Geometry: final body of the model. Coordinates: model frame, mm. A direction names the side the tool comes from. Round coordinates to 2 decimals unless told otherwise and drop trailing zeros. Loops run counter-clockwise (first coordinate to the right, second up) from the corner with the lowest first, then second, coordinate; pieces in that order, holes last. Notation, with made-up numbers: (-19.75, 70) -> (26.25, 70) arc R22 ccw to (26.25, 99) -> close; hole circle Ø10 at (-6.5, 37). An arc over 180 degrees is marked (long way). Answer in a Markdown table with one row per item.
```python
from build123d import *

# Parameters (mm, degrees)
ESQUISSE1_R             = 1.1
BOSS_EXTRU_1_DEPTH      = 2.1
ESQUISSE2_R             = 3.35
ESQUISSE2_R_2           = 2.55
BOSS_EXTRU_2_DEPTH      = 0.2
ENL_V_START             = -0.8
ESQUISSE9_R             = 2.55
ENL_V_MAT_EXTRU_4_DEPTH = 0.8
BOSS_EXTRU_3_START      = 2.5
ESQUISSE5_R             = 3.35
ESQUISSE5_R_2           = 2.55
BOSS_EXTRU_3_DEPTH      = 4.8
ENL_V_MAT_EXTRU_3_REACH = 26.785
ESQUISSE7_R             = 0.5


with BuildPart() as part:
    # Esquisse1 → Boss.-Extru.1 (new body)
    with BuildSketch(Plane(origin=(0, 0, 0), x_dir=(1, 0, 0), z_dir=(0, 1, 0))):
        with BuildLine():
            Line((8.85, 1.9), (-5.55, 3.193286234))
            Line((-5.55, 3.193286234), (-5.55, 6.3))
            ThreePointArc((-5.55, 6.3), (-7.4, 8.15), (-9.25, 6.3))
            Line((-9.25, 6.3), (-9.25, 2.95))
            Line((-9.25, 2.95), (-21.15, 1.8))
            ThreePointArc((-21.15, 1.8), (-22.95, 0), (-21.15, -1.8))
            Line((-21.15, -1.8), (-9.25, -2.95))
            Line((-9.25, -2.95), (-9.25, -6.3))
            ThreePointArc((-9.25, -6.3), (-7.4, -8.15), (-5.55, -6.3))
            Line((-5.55, -6.3), (-5.55, -3.193286234))
            Line((-5.55, -3.193286234), (8.85, -1.9))
            ThreePointArc((8.85, -1.9), (10.75, 0), (8.85, 1.9))
        make_face()
        with Locations(Location((-7.4, 0, 0), (0, 0, 270))):
            Circle(ESQUISSE1_R, mode=Mode.SUBTRACT)
    extrude(amount=BOSS_EXTRU_1_DEPTH)

    # Esquisse2 → Boss.-Extru.2 (add)
    with BuildSketch(Plane(origin=(0, 2.1, 0), x_dir=(1, 0, 0), z_dir=(0, 1, 0))):
        with Locations(Location((-7.4, 0, 0), (0, 0, 270))):
            Circle(ESQUISSE2_R)
        with Locations(Location((-7.4, 0, 0), (0, 0, 270))):
            Circle(ESQUISSE2_R_2, mode=Mode.SUBTRACT)
    extrude(amount=BOSS_EXTRU_2_DEPTH)

    # Esquisse9 → Enlèv. mat.-Extru.4 (cut)
    with BuildSketch(Plane(origin=(0, 2.3, 0), x_dir=(1, 0, 0), z_dir=(0, 1, 0)).offset(ENL_V_START)):
        with Locations(Location((-7.4, 0, 0), (0, 0, 270))):
            Circle(ESQUISSE9_R)
    extrude(amount=ENL_V_MAT_EXTRU_4_DEPTH, mode=Mode.SUBTRACT)

    # Esquisse5 → Boss.-Extru.3 (add)
    with BuildSketch(Plane.XZ.offset(BOSS_EXTRU_3_START)):
        with Locations(Location((-7.4, 0, 0), (0, 0, 90))):
            Circle(ESQUISSE5_R)
        with Locations(Location((-7.4, 0, 0), (0, 0, 90))):
            Circle(ESQUISSE5_R_2, mode=Mode.SUBTRACT)
    extrude(amount=-BOSS_EXTRU_3_DEPTH)

    # Esquisse7 → Enlèv. mat.-Extru.3 (cut, up to next)
    with BuildSketch(Plane(origin=(0, 2.1, 0), x_dir=(1, 0, 0), z_dir=(0, 1, 0)), mode=Mode.PRIVATE) as enl_v_mat_extru_3_sk1:
        with Locations(Location((-7.4, 4.35, 0), (0, 0, 270))):
            Circle(ESQUISSE7_R)
    enl_v_mat_extru_3_tool1 = extrude(enl_v_mat_extru_3_sk1.sketch, amount=-ENL_V_MAT_EXTRU_3_REACH, mode=Mode.PRIVATE) & part.part
    # Esquisse7 → Enlèv. mat.-Extru.3 (cut, up to next)
    with BuildSketch(Plane(origin=(0, 2.1, 0), x_dir=(1, 0, 0), z_dir=(0, 1, 0)), mode=Mode.PRIVATE) as enl_v_mat_extru_3_sk2:
        with Locations(Location((-7.4, 6.65, 0), (0, 0, 270))):
            Circle(ESQUISSE7_R)
    enl_v_mat_extru_3_tool2 = extrude(enl_v_mat_extru_3_sk2.sketch, amount=-ENL_V_MAT_EXTRU_3_REACH, mode=Mode.PRIVATE) & part.part
    # Esquisse7 → Enlèv. mat.-Extru.3 (cut, up to next)
    with BuildSketch(Plane(origin=(0, 2.1, 0), x_dir=(1, 0, 0), z_dir=(0, 1, 0)), mode=Mode.PRIVATE) as enl_v_mat_extru_3_sk3:
        with Locations(Location((-2.55, 0, 0), (0, 0, 270))):
            Circle(ESQUISSE7_R)
    enl_v_mat_extru_3_tool3 = extrude(enl_v_mat_extru_3_sk3.sketch, amount=-ENL_V_MAT_EXTRU_3_REACH, mode=Mode.PRIVATE) & part.part
    # Esquisse7 → Enlèv. mat.-Extru.3 (cut, up to next)
    with BuildSketch(Plane(origin=(0, 2.1, 0), x_dir=(1, 0, 0), z_dir=(0, 1, 0)), mode=Mode.PRIVATE) as enl_v_mat_extru_3_sk4:
        with Locations(Location((-0.6, 0, 0), (0, 0, 270))):
            Circle(ESQUISSE7_R)
    enl_v_mat_extru_3_tool4 = extrude(enl_v_mat_extru_3_sk4.sketch, amount=-ENL_V_MAT_EXTRU_3_REACH, mode=Mode.PRIVATE) & part.part
    # Esquisse7 → Enlèv. mat.-Extru.3 (cut, up to next)
    with BuildSketch(Plane(origin=(0, 2.1, 0), x_dir=(1, 0, 0), z_dir=(0, 1, 0)), mode=Mode.PRIVATE) as enl_v_mat_extru_3_sk5:
        with Locations(Location((1.35, 0, 0), (0, 0, 270))):
            Circle(ESQUISSE7_R)
    enl_v_mat_extru_3_tool5 = extrude(enl_v_mat_extru_3_sk5.sketch, amount=-ENL_V_MAT_EXTRU_3_REACH, mode=Mode.PRIVATE) & part.part
    # Esquisse7 → Enlèv. mat.-Extru.3 (cut, up to next)
    with BuildSketch(Plane(origin=(0, 2.1, 0), x_dir=(1, 0, 0), z_dir=(0, 1, 0)), mode=Mode.PRIVATE) as enl_v_mat_extru_3_sk6:
        with Locations(Location((3.3, 0, 0), (0, 0, 270))):
            Circle(ESQUISSE7_R)
    enl_v_mat_extru_3_tool6 = extrude(enl_v_mat_extru_3_sk6.sketch, amount=-ENL_V_MAT_EXTRU_3_REACH, mode=Mode.PRIVATE) & part.part
    # Esquisse7 → Enlèv. mat.-Extru.3 (cut, up to next)
    with BuildSketch(Plane(origin=(0, 2.1, 0), x_dir=(1, 0, 0), z_dir=(0, 1, 0)), mode=Mode.PRIVATE) as enl_v_mat_extru_3_sk7:
        with Locations(Location((5.25, 0, 0), (0, 0, 270))):
            Circle(ESQUISSE7_R)
    enl_v_mat_extru_3_tool7 = extrude(enl_v_mat_extru_3_sk7.sketch, amount=-ENL_V_MAT_EXTRU_3_REACH, mode=Mode.PRIVATE) & part.part
    # Esquisse7 → Enlèv. mat.-Extru.3 (cut, up to next)
    with BuildSketch(Plane(origin=(0, 2.1, 0), x_dir=(1, 0, 0), z_dir=(0, 1, 0)), mode=Mode.PRIVATE) as enl_v_mat_extru_3_sk8:
        with Locations(Location((7.2, 0, 0), (0, 0, 270))):
            Circle(ESQUISSE7_R)
    enl_v_mat_extru_3_tool8 = extrude(enl_v_mat_extru_3_sk8.sketch, amount=-ENL_V_MAT_EXTRU_3_REACH, mode=Mode.PRIVATE) & part.part
    # Esquisse7 → Enlèv. mat.-Extru.3 (cut, up to next)
    with BuildSketch(Plane(origin=(0, 2.1, 0), x_dir=(1, 0, 0), z_dir=(0, 1, 0)), mode=Mode.PRIVATE) as enl_v_mat_extru_3_sk9:
        with Locations(Location((9.15, 0, 0), (0, 0, 270))):
            Circle(ESQUISSE7_R)
    enl_v_mat_extru_3_tool9 = extrude(enl_v_mat_extru_3_sk9.sketch, amount=-ENL_V_MAT_EXTRU_3_REACH, mode=Mode.PRIVATE) & part.part
    # Esquisse7 → Enlèv. mat.-Extru.3 (cut, up to next)
    with BuildSketch(Plane(origin=(0, 2.1, 0), x_dir=(1, 0, 0), z_dir=(0, 1, 0)), mode=Mode.PRIVATE) as enl_v_mat_extru_3_sk10:
        with Locations(Location((-7.4, -6.65, 0), (0, 0, 270))):
            Circle(ESQUISSE7_R)
    enl_v_mat_extru_3_tool10 = extrude(enl_v_mat_extru_3_sk10.sketch, amount=-ENL_V_MAT_EXTRU_3_REACH, mode=Mode.PRIVATE) & part.part
    # Esquisse7 → Enlèv. mat.-Extru.3 (cut, up to next)
    with BuildSketch(Plane(origin=(0, 2.1, 0), x_dir=(1, 0, 0), z_dir=(0, 1, 0)), mode=Mode.PRIVATE) as enl_v_mat_extru_3_sk11:
        with Locations(Location((-7.4, -4.35, 0), (0, 0, 270))):
            Circle(ESQUISSE7_R)
    enl_v_mat_extru_3_tool11 = extrude(enl_v_mat_extru_3_sk11.sketch, amount=-ENL_V_MAT_EXTRU_3_REACH, mode=Mode.PRIVATE) & part.part
    # Esquisse7 → Enlèv. mat.-Extru.3 (cut, up to next)
    with BuildSketch(Plane(origin=(0, 2.1, 0), x_dir=(1, 0, 0), z_dir=(0, 1, 0)), mode=Mode.PRIVATE) as enl_v_mat_extru_3_sk12:
        with Locations(Location((-11.75, 0, 0), (0, 0, 270))):
            Circle(ESQUISSE7_R)
    enl_v_mat_extru_3_tool12 = extrude(enl_v_mat_extru_3_sk12.sketch, amount=-ENL_V_MAT_EXTRU_3_REACH, mode=Mode.PRIVATE) & part.part
    # Esquisse7 → Enlèv. mat.-Extru.3 (cut, up to next)
    with BuildSketch(Plane(origin=(0, 2.1, 0), x_dir=(1, 0, 0), z_dir=(0, 1, 0)), mode=Mode.PRIVATE) as enl_v_mat_extru_3_sk13:
        with Locations(Location((-13.67, 0, 0), (0, 0, 270))):
            Circle(ESQUISSE7_R)
    enl_v_mat_extru_3_tool13 = extrude(enl_v_mat_extru_3_sk13.sketch, amount=-ENL_V_MAT_EXTRU_3_REACH, mode=Mode.PRIVATE) & part.part
    # Esquisse7 → Enlèv. mat.-Extru.3 (cut, up to next)
    with BuildSketch(Plane(origin=(0, 2.1, 0), x_dir=(1, 0, 0), z_dir=(0, 1, 0)), mode=Mode.PRIVATE) as enl_v_mat_extru_3_sk14:
        with Locations(Location((-15.59, 0, 0), (0, 0, 270))):
            Circle(ESQUISSE7_R)
    enl_v_mat_extru_3_tool14 = extrude(enl_v_mat_extru_3_sk14.sketch, amount=-ENL_V_MAT_EXTRU_3_REACH, mode=Mode.PRIVATE) & part.part
    # Esquisse7 → Enlèv. mat.-Extru.3 (cut, up to next)
    with BuildSketch(Plane(origin=(0, 2.1, 0), x_dir=(1, 0, 0), z_dir=(0, 1, 0)), mode=Mode.PRIVATE) as enl_v_mat_extru_3_sk15:
        with Locations(Location((-17.51, 0, 0), (0, 0, 270))):
            Circle(ESQUISSE7_R)
    enl_v_mat_extru_3_tool15 = extrude(enl_v_mat_extru_3_sk15.sketch, amount=-ENL_V_MAT_EXTRU_3_REACH, mode=Mode.PRIVATE) & part.part
    # Esquisse7 → Enlèv. mat.-Extru.3 (cut, up to next)
    with BuildSketch(Plane(origin=(0, 2.1, 0), x_dir=(1, 0, 0), z_dir=(0, 1, 0)), mode=Mode.PRIVATE) as enl_v_mat_extru_3_sk16:
        with Locations(Location((-19.43, 0, 0), (0, 0, 270))):
            Circle(ESQUISSE7_R)
    enl_v_mat_extru_3_tool16 = extrude(enl_v_mat_extru_3_sk16.sketch, amount=-ENL_V_MAT_EXTRU_3_REACH, mode=Mode.PRIVATE) & part.part
    # Esquisse7 → Enlèv. mat.-Extru.3 (cut, up to next)
    with BuildSketch(Plane(origin=(0, 2.1, 0), x_dir=(1, 0, 0), z_dir=(0, 1, 0)), mode=Mode.PRIVATE) as enl_v_mat_extru_3_sk17:
        with Locations(Location((-21.35, 0, 0), (0, 0, 270))):
            Circle(ESQUISSE7_R)
    enl_v_mat_extru_3_tool17 = extrude(enl_v_mat_extru_3_sk17.sketch, amount=-ENL_V_MAT_EXTRU_3_REACH, mode=Mode.PRIVATE) & part.part
    add(enl_v_mat_extru_3_tool1.solids().sort_by_distance((-7.4, 2.1, -4.35))[0], mode=Mode.SUBTRACT)
    add(enl_v_mat_extru_3_tool2.solids().sort_by_distance((-7.4, 2.1, -6.65))[0], mode=Mode.SUBTRACT)
    add(enl_v_mat_extru_3_tool3.solids().sort_by_distance((-2.55, 2.1, 0))[0], mode=Mode.SUBTRACT)
    add(enl_v_mat_extru_3_tool4.solids().sort_by_distance((-0.6, 2.1, 0))[0], mode=Mode.SUBTRACT)
    add(enl_v_mat_extru_3_tool5.solids().sort_by_distance((1.35, 2.1, 0))[0], mode=Mode.SUBTRACT)
    add(enl_v_mat_extru_3_tool6.solids().sort_by_distance((3.3, 2.1, 0))[0], mode=Mode.SUBTRACT)
    add(enl_v_mat_extru_3_tool7.solids().sort_by_distance((5.25, 2.1, 0))[0], mode=Mode.SUBTRACT)
    add(enl_v_mat_extru_3_tool8.solids().sort_by_distance((7.2, 2.1, 0))[0], mode=Mode.SUBTRACT)
    add(enl_v_mat_extru_3_tool9.solids().sort_by_distance((9.15, 2.1, 0))[0], mode=Mode.SUBTRACT)
    add(enl_v_mat_extru_3_tool10.solids().sort_by_distance((-7.4, 2.1, 6.65))[0], mode=Mode.SUBTRACT)
    add(enl_v_mat_extru_3_tool11.solids().sort_by_distance((-7.4, 2.1, 4.35))[0], mode=Mode.SUBTRACT)
    add(enl_v_mat_extru_3_tool12.solids().sort_by_distance((-11.75, 2.1, 0))[0], mode=Mode.SUBTRACT)
    add(enl_v_mat_extru_3_tool13.solids().sort_by_distance((-13.67, 2.1, 0))[0], mode=Mode.SUBTRACT)
    add(enl_v_mat_extru_3_tool14.solids().sort_by_distance((-15.59, 2.1, 0))[0], mode=Mode.SUBTRACT)
    add(enl_v_mat_extru_3_tool15.solids().sort_by_distance((-17.51, 2.1, 0))[0], mode=Mode.SUBTRACT)
    add(enl_v_mat_extru_3_tool16.solids().sort_by_distance((-19.43, 2.1, 0))[0], mode=Mode.SUBTRACT)
    add(enl_v_mat_extru_3_tool17.solids().sort_by_distance((-21.35, 2.1, 0))[0], mode=Mode.SUBTRACT)


solid = part.part
```
Item 1: Section query D-D, the plane y = -2.05. Output: boundary loops of the cut face in (x, z), and give its area (3 significant figures).
Ans:
| item | result |
|---|---|
| outline | circle Ø6.7 at (-7.4, 0); hole circle Ø5.1 at (-7.4, 0) |
| area | 14.8 mm2 |
Item 2: Section query A-A, the plane z = 4.35. Output: boundary loops of the cut face in (x, y), and give its area (3 significant figures).
Ans:
| item | result |
|---|---|
| outline | (-9.25, 0) -> (-7.9, 0) -> (-7.9, 2.1) -> (-9.25, 2.1) -> close; (-6.9, 0) -> (-5.55, 0) -> (-5.55, 2.1) -> (-6.9, 2.1) -> close |
| area | 5.67 mm2 |
Item 3: Section query C-C, the plane y = 0.85. State how many separate pieces and enclosed holes the cut face has, and give its area (3 significant figures).
Ans:
| item | result |
|---|---|
| separate pieces | 1 |
| enclosed holes | 18 |
| area | 181 mm2 |
Item 4: First-contact query: P1, Ø0.6, axis at y = 1, z = 5, coming from the -X side; P2, Ø4.5, axis at x = -7.4, z = 0, coming from the -Y side; P3, Ø4.5, axis at x = -7.4, z = 0, coming from the +Y side. Flat tips, straight axial feed; report the tip coordinate or a pass-through.
Ans:
| item | result |
|---|---|
| P1 | x = -9.25 |
| P2 | y = 0 |
| P3 | y = 1.5 |
Item 5: Ray query, L1, parallel to Z at x = -8, y = -0.55; L2, parallel to X at y = 1.6, z = -5; L3, parallel to X at y = 1.3, z = 4.35. Return the intervals inside material, ascending.
Ans:
| item | result |
|---|---|
| L1 | -3.3 to -2.48, 2.48 to 3.3 |
| L2 | -9.25 to -5.55 |
| L3 | -9.25 to -7.9, -6.9 to -5.55 |
Item 6: Set-up query: faces 1 (the cylindrical face through (-16.078, 1.065, -0.108)), 2 (the flat face through (-6, 1.5, 0)). Return all of +Z, -Z, +X, -X, +Y, -Y with unobstructed straight access to the full face (end or side cutting, diameter ignored); none if empty.
Ans:
| item | result |
|---|---|
| face 1 | +Y, -Y |
| face 2 | +Y |
Item 7: Mould query, pull axis X, two halves, no side actions, for faces 3 (the cylindrical face through (5.746, 1.065, -0.065)), 4 (the cylindrical face through (-22.95, 1.04, -0.04)), 5 (the flat face through (-10, 2.3, -1)). Classes: released by +X, released by -X, zero draft, split by the parting line, or undercut.
Ans:
| item | result |
|---|---|
| face 3 | undercut |
| face 4 | released by -X |
| face 5 | zero draft |
Item 8: Section query B-B, the plane x = -13.67. Output: boundary loops of the cut face in (y, z), and give its area (3 significant figures).
Ans:
| item | result |
|---|---|
| outline | (0, -2.52) -> (2.1, -2.52) -> (2.1, -0.5) -> (0, -0.5) -> close; (0, 0.5) -> (2.1, 0.5) -> (2.1, 2.52) -> (0, 2.52) -> close |
| area | 8.50 mm2 |
